Can you work these out from the model? Positions are in its coordinate system, mm. A direction names the side the tool comes from. Coordinates: 2 decimals unless noted, no trailing zeros. Loops run counter-clockwise (first coordinate to the right, second up) from the corner with the lowest first, then second, coordinate; pieces in that order, holes last.
```python
from build123d import *

# Parameters (mm, degrees)
SKETCH1_R           = 2.25
BOSS_EXTRUDE1_DEPTH = 10


with BuildPart() as part:
    # Sketch1 → Boss-Extrude1 (new body)
    with BuildSketch(Plane.XY):
        with BuildLine():
            Line((15, 19.25), (-15, 19.25))
            Line((-15, 19.25), (-30, 19.25))
            Line((-30, 19.25), (-40, 19.25))
            ThreePointArc((-40, 19.25), (-43.535533906, 17.785533906), (-45, 14.25))
            Line((-45, 14.25), (-45, -14.25))
            ThreePointArc((-45, -14.25), (-43.535533906, -17.785533906), (-40, -19.25))
            Line((-40, -19.25), (-30, -19.25))
            Line((-30, -19.25), (-15, -19.25))
            Line((-15, -19.25), (-8.5, -19.25))
            Line((-8.5, -19.25), (-8.5, -16.75))
            Line((-8.5, -16.75), (-8.5, -11.437329234))
            ThreePointArc((-8.5, -11.437329234), (0, 14.25), (8.5, -11.437329234))
            Line((8.5, -11.437329234), (8.5, -16.75))
            Line((8.5, -16.75), (8.5, -19.25))
            Line((8.5, -19.25), (15, -19.25))
            Line((15, -19.25), (30, -19.25))
            Line((30, -19.25), (40, -19.25))
            ThreePointArc((40, -19.25), (43.535533906, -17.785533906), (45, -14.25))
            Line((45, -14.25), (45, 14.25))
            ThreePointArc((45, 14.25), (43.535533906, 17.785533906), (40, 19.25))
            Line((40, 19.25), (30, 19.25))
            Line((30, 19.25), (15, 19.25))
        make_face()
        with Locations((-15, -15)):
            Circle(SKETCH1_R, mode=Mode.SUBTRACT)
        with Locations((15, -15)):
            Circle(SKETCH1_R, mode=Mode.SUBTRACT)
        with Locations((-15, 15)):
            Circle(SKETCH1_R, mode=Mode.SUBTRACT)
        with Locations((15, 15)):
            Circle(SKETCH1_R, mode=Mode.SUBTRACT)
    extrude(amount=BOSS_EXTRUDE1_DEPTH)


solid = part.part
```
Item 1: Suppose I cut it at C-C, the plane x = 0. Please give me the cut outline in (y, z).
Results are:
outline: (14.25, 0) - (19.25, 0) - (19.25, 10) - (14.25, 10) - close
Item 2: Suppose I cut it at A-A, the plane y = 11.5. Please give me the cut outline in (x, z).
Results are:
outline: (-45, 0) - (-8.42, 0) - (-8.42, 10) - (-45, 10) - close; (8.42, 0) - (45, 0) - (45, 10) - (8.42, 10) - close
Item 3: I need wall thicknesses on line 1 along Y through (x, z) = (15, 5.75); line 2 along X through (y, z) = (0, 5); line 3 along X through (y, z) = (9, 2.5). Which ranges of each line are inside material? Lowest first, please.
Results are:
line 1: y = -19.25 to -17.25, -12.75 to 12.75, 17.25 to 19.25
line 2: x = -45 to -14.25, 14.25 to 45
line 3: x = -45 to -11.05, 11.05 to 45
Item 4: Suppose I cut it at B-B, the plane z = 4.5. Please give me the cut outline in (x, y), plus the area to 3 significant figures.
Results are:
outline: (-45, -14.25) arc R5 ccw to (-40, -19.25) - (-8.5, -19.25) - (-8.5, -11.44) arc R14.25 cw (long way) to (8.5, -11.44) - (8.5, -19.25) - (40, -19.25) arc R5 ccw to (45, -14.25) - (45, 14.25) arc R5 ccw to (40, 19.25) - (-40, 19.25) arc R5 ccw to (-45, 14.25) - close; hole circle Ø4.5 at (-15, -15); hole circle Ø4.5 at (-15, 15); hole circle Ø4.5 at (15, -15); hole circle Ø4.5 at (15, 15)
area: 2,640 mm2
Item 5: On a 3-axis mill with a long thin cutter (end or side, diameter ignored), from which of +Z, -Z, +X, -X, +Y, -Y can I reach the whole of each face in a straight line? I mean faces 4 (the face through (-11, 13, 0)), 5 (the face through (-8.5, -15, 5)). Say none if no direction works.
Results are:
face 4: -Z, +X, -X, +Y, -Y
face 5: +Z, -Z, -Y
Item 6: Suppose I cut it at D-D, the plane y = 0. Please give me the cut outline in (x, z).
Results are:
outline: (-45, 0) - (-14.25, 0) - (-14.25, 10) - (-45, 10) - close; (14.25, 0) - (45, 0) - (45, 10) - (14.25, 10) - close
Item 7: We'd pull the mould along X, two halves only. Please class faces 1 (the face through (43.5, -17.82, 4.93)), 2 (the face through (-12.92, -15.86, 4.93)), 3 (the face through (1, 19.25, 5)): +X half, -X half, draft (parallel to the pull), parting line (faces both ways), or undercut.
Results are:
face 1: +X half
face 2: undercut
face 3: draft
